Input: part model. Units: mm. Frame: model coordinates. Coordinates: 2 decimals unless noted, no trailing zeros. Loops run counter-clockwise (first coordinate to the right, second up) from the corner with the lowest first, then second, coordinate; pieces in that order, holes last. Notation, with made-up numbers: M 20.25,33.5 L 26.25,33.5 A25 cw 26.25,58.5 Z; hole C -12,5 d5. An arc over 180 degrees is marked long. Use a Markdown table: item, result. Add a question column.
1. Section A-A on z = 181.5. Output: boundary loops of the cut face in (x, y), then the cut area to 3 significant figures.
2. Pin query (flat end, axial travel): pin 1 (6 mm diameter, centred on y = 51.5, z = -46, fed in from -X); pin 2 (12 mm diameter, centred on y = 32, z = 223.5, fed in from -X). Return the tip coordinate at first contact, or that it passes through.
3. Line query: L1, parallel to X at y = 12, z = -255; L2, parallel to X at y = 8, z = 153; L3, parallel to Z at x = -89.5, y = 7.5. Output: solid intervals per line, ascending. Write a range as [from, to].
```python
from build123d import *

# Parameters (mm, degrees)
BOSS_EXTRUDE1_DEPTH = 296
FILLET1_R           = 10


with BuildPart() as part:
    # Sketch1 → Boss-Extrude1 (new, symmetric)
    with BuildSketch(Plane.XY):
        Polygon((0, 0), (-996, 0), (-938.450475902, 75), (0, 75), align=None)
    extrude(amount=BOSS_EXTRUDE1_DEPTH, both=True)

    # Fillet1
    fillet1_edges = [part.edges().sort_by_distance(p)[0] for p in [
        (-967.225237951, 37.5, 296),
        (-498, 0, 296),
        (0, 37.5, 296),
        (-498, 0, -296),
        (-967.225237951, 37.5, -296),
        (-469.225237951, 75, -296),
        (0, 37.5, -296),
        (0, 0, 0),
        (-996, 0, 0),
        (-938.450475902, 75, 0),
        (0, 75, 0),
        (-469.225237951, 75, 296),
    ]]
    fillet(fillet1_edges, radius=FILLET1_R)


solid = part.part
```
Answers below:
| question | item | result |
|---|---|---|
| 1 | outline | M -983.66,16.09 A10 ccw -975.72,0 L -10,0 A10 ccw 0,10 L 0,65 A10 ccw -10,75 L -933.52,75 A10 ccw -941.45,71.09 Z |
| 1 | area | 72,400 mm² |
| 2 | pin 1 | stops at x = -958.78 |
| 2 | pin 2 | stops at x = -976.05 |
| 3 | L1 | x = [-985.52, 0] |
| 3 | L2 | x = [-985.52, -0.2] |
| 3 | L3 | z = [-295.68, 295.68] |
